Read the model definition and answer for the solid it produces. Units are mm, in the model's axes. A direction names the side the tool comes from. Coordinates: 2 decimals unless noted, no trailing zeros. Loops run counter-clockwise (first coordinate to the right, second up) from the corner with the lowest first, then second, coordinate; pieces in that order, holes last.
Q1. Section B-B (z = 9) is taken. Give the vertices of the cut face in (x, y).
Q2. Section D-D (z = 63) is taken. Give the vertices of the cut face in (x, y), then the cut area to 3 significant figures.
Q3. The mould has two halves that part along X. Classify faces 1 (the face through (24, 2, 1.2)), 2 (the face through (0, 2, 35)), 3 (the face through (24, 2, 0)): pulls with the +X half, pulls with the -X half, needs draft (parallel to the pull), parting line crosses it, or undercut.
Q4. Which of the six approach directions +Z, -Z, +X, -X, +Y, -Y give full straight-line access (tool end or side, diameter ignored) to faces 4 (the face through (0.6, 2, 37)), 5 (the face through (23.8, 4.4, 71.2)), 6 (the face through (23.425, 0.296, 58.703))?
Q5. Section C-C (y = 3.3) is taken. Give the vertices of the cut face in (x, z), then the cut area to 3 significant figures.
Q6. Straight lines are drawn through the part: line 1 (Y direction, x = 41.5, z = 8); line 2 (X direction, y = 3.45, z = 39.5); line 3 (Z direction, x = 23.5, y = 1.7). For each, find the intervals that lie inside material, in ascending order.
Q7. Section A-A (x = 38) is taken. Give the vertices of the cut face in (y, z), then the cut area to 3 significant figures.
from build123d import *

# Parameters (mm, degrees)
SKETCH_W        = 47.8
SKETCH_H        = 4.8
PAD_DEPTH       = 71.2
SKETCH001_W     = 46.6
SKETCH001_H     = 3.6
POCKET_DEPTH    = 70
SKETCH002_R     = 12.5
POCKET001_DEPTH = 0.6


with BuildPart() as part:
    # Sketch → Pad (new body)
    with BuildSketch(Plane.XY):
        with Locations((23.9, 2.4)):
            Rectangle(SKETCH_W, SKETCH_H)
    extrude(amount=PAD_DEPTH)

    # Sketch001 (on Face6 of Pad) → Pocket (cut)
    with BuildSketch(Plane.XY.offset(71.2)):
        with Locations((23.9, 2.4)):
            Rectangle(SKETCH001_W, SKETCH001_H)
    extrude(amount=-POCKET_DEPTH, mode=Mode.SUBTRACT)

    # Sketch002 (on Face6 of Pocket) → Pocket001 (cut)
    with BuildSketch(Plane.XZ):
        with Locations((23.7, 71.2)):
            Circle(SKETCH002_R)
    extrude(amount=-POCKET001_DEPTH, mode=Mode.SUBTRACT)


solid = part.part
Numbers:
1. outline: (0, 0) - (47.8, 0) - (47.8, 4.8) - (0, 4.8) - close; hole (0.6, 0.6) - (47.2, 0.6) - (47.2, 4.2) - (0.6, 4.2) - close
2. outline: (0, 0) - (14.27, 0) - (14.27, 0.6) - (0.6, 0.6) - (0.6, 4.2) - (47.2, 4.2) - (47.2, 0.6) - (33.13, 0.6) - (33.13, 0) - (47.8, 0) - (47.8, 4.8) - (0, 4.8) - close
2. area: 50.4 mm2
3. face 1: undercut
3. face 2: pulls with the -X half
3. face 3: needs draft
4. face 4: +Z
4. face 5: +Z, +X, -X, +Y, -Y
4. face 6: +Z, -Y
5. outline: (0, 0) - (47.8, 0) - (47.8, 71.2) - (47.2, 71.2) - (47.2, 1.2) - (0.6, 1.2) - (0.6, 71.2) - (0, 71.2) - close
5. area: 141 mm2
6. line 1: y = 0 to 0.6, 4.2 to 4.8
6. line 2: x = 0 to 0.6, 47.2 to 47.8
6. line 3: z = 0 to 1.2
7. outline: (0, 0) - (4.8, 0) - (4.8, 71.2) - (4.2, 71.2) - (4.2, 1.2) - (0.6, 1.2) - (0.6, 71.2) - (0, 71.2) - close
7. area: 89.8 mm2
